Geometry: final body of the model. Coordinates: model frame, mm. A direction names the side the tool comes from. Give positions to 0.01 mm unless a question says otherwise; leave off trailing zeros. Order: outer loops, then holes, each group sorted by start corner. A loop starts at its lowest first (then second) coordinate and runs counter-clockwise, first axis right, second up. Notation, with made-up numbers: (-15.5, 0) -> (13.5, 0) arc R33 cw to (13.5, 32) -> close; hole circle Ø11 at (-40, 33.5). An arc over 180 degrees is marked (long way). Answer in a Markdown table with one row per item. Add a question column.
Q1. Line query: line 1 along Y through (x, z) = (-23, 0); line 2 along X through (y, z) = (28.5, 13.5); line 3 along Y through (x, z) = (-21.5, -3.5). Output: solid intervals per line, ascending. Write a range as from..to.
Q2. Contact query for flat-ended pins moving along their axis: P1, Ø10.5, axis at y = 55, z = 0.25, coming from the -X side; P2, Ø4.5, axis at x = 1, y = 52, coming from the -Z side; P3, Ø3, axis at x = 22.5, y = 14.5, coming from the -Z side; P4, Ø5.5, axis at y = 35.79, z = 0.25, coming from the +X side. Output: stop coordinate, or through.
Q3. Cut plane D-D on x = -10. Return the cut outline in (y, z), and give its area (3 significant figures).
Q4. Cut plane A-A on x = 0. Return the cut outline in (y, z), and give its area (3 significant figures).
Q5. Cut plane C-C on z = -16. Return the cut outline in (x, y).
Q6. Cut plane B-B on y = 20. Return the cut outline in (x, z), and give its area (3 significant figures).
Q7. Pull-direction query (Z, two-part tool) for faces 6 (the face through (-24.278, 48.132, -1.275)), 7 (the face through (23, 26.5, -7)), 8 (the face through (23, 47, -19.75)); classes: +Z half, -Z half, draft (parallel to the pull), parting line (faces both ways), or undercut.
Q8. Set-up query: faces 1 (the face through (22.25, 55, 5)), 2 (the face through (20.25, 42, 0)), 3 (the face through (-22.25, 55, 5)), 4 (the face through (23.21, 25, 8.82)), 5 (the face through (0, 51, 22.35)). Return all of +Z, -Z, +X, -X, +Y, -Y with unobstructed straight access to the full face (end or side cutting, diameter ignored); none if empty.
from build123d import *

# Parameters (mm, degrees)
BOSS_EXTRUDE1_DEPTH           = 70
SKETCH8_R                     = 4.5
CUT_EXTRUDE4_DEPTH            = 53.5
SKETCH10_R                    = 7.035
CUT_EXTRUDE5_DEPTH            = 4
FILLET13_R                    = 1
M8_CLEARANCE_HOLE1_AT_2_COUNT = 2
M8_CLEARANCE_HOLE1_AT_2_PITCH = 24.109474775
CUT_EXTRUDE6_REACH            = 54.5
SKETCH21_W                    = 30
SKETCH21_H                    = 26.5
M8_CLEARANCE_HOLE2_D          = 9
FILLET14_R                    = 5
SKETCH24_W                    = 10
SKETCH24_H                    = 38
CUT_EXTRUDE7_DEPTH            = 2.1
FILLET15_R                    = 0.5


with BuildPart() as part:
    # Sketch1 → Boss-Extrude1 (new body)
    with BuildSketch(Plane(origin=(0, 0, 0), x_dir=(1, 0, 0), z_dir=(0, 1, 0))):
        Polygon((-26.25, -26.25), (26.25, -26.25), (26.25, 19.75), (20.25, 19.75), (20.25, -20.25), (-20.25, -20.25), (-20.25, 19.75), (-26.25, 19.75), align=None)
    extrude(amount=BOSS_EXTRUDE1_DEPTH)

    # Sketch8 → Cut-Extrude4 (cut, through all)
    with BuildSketch(Plane(origin=(26.25, 0, 0), x_dir=(0, 0, -1), z_dir=(1, 0, 0))):
        with Locations((-0.25, 55)):
            Circle(SKETCH8_R)
    extrude(amount=-CUT_EXTRUDE4_DEPTH, mode=Mode.SUBTRACT)

    # Sketch10 → Cut-Extrude5 (cut)
    with BuildSketch(Plane.ZY.offset(26.25)):
        with Locations((0.25, 55)):
            Circle(SKETCH10_R)
    cut_extrude5 = extrude(amount=-CUT_EXTRUDE5_DEPTH, mode=Mode.SUBTRACT)

    # Mirror1: Cut-Extrude5 across plane
    add(cut_extrude5.mirror(Plane(origin=(0, 0, 0), x_dir=(0, 0, 1), z_dir=(1, 0, 0))), mode=Mode.SUBTRACT)

    # Fillet13
    fillet13_edges = [part.edges().sort_by_distance(p)[0] for p in [
        (26.25, 0, 3.25),
        (0, 0, 26.25),
        (0, 70, 20.25),
        (-26.25, 0, 3.25),
        (-23.25, 0, -19.75),
        (-20.25, 0, 0.25),
        (0, 0, 20.25),
        (20.25, 0, 0.25),
        (-20.25, 70, 0.25),
        (20.25, 35, -19.75),
        (26.25, 35, -19.75),
        (26.25, 35, 26.25),
        (-26.25, 35, 26.25),
        (-26.25, 35, -19.75),
        (-20.25, 35, -19.75),
        (-23.25, 70, -19.75),
        (-26.25, 70, 3.25),
        (0, 70, 26.25),
        (26.25, 70, 3.25),
        (23.25, 70, -19.75),
        (20.25, 70, 0.25),
        (23.25, 0, -19.75),
    ]]
    fillet(fillet13_edges, radius=FILLET13_R)

    # Sketch18 → M8 Clearance Hole1 (revolve, cut)
    with BuildSketch(Plane(origin=(-20.25, 35.786178525, 0.25), x_dir=(0, 0, -1), z_dir=(0, 1, 0))):
        Polygon((0, 0), (0, 15.703872786), (4.5, 13), (4.5, 0.025), (4.525, 0), align=None)
    m8_clearance_hole1 = revolve(axis=Axis((-13.9, 35.786178525, 0.25), (-1, 0, 0)), mode=Mode.SUBTRACT)

    # M8 Clearance Hole1 at 2: M8 Clearance Hole1 ×2
    with Locations(*[(0, -i * M8_CLEARANCE_HOLE1_AT_2_PITCH, 0) for i in range(1, M8_CLEARANCE_HOLE1_AT_2_COUNT)]):
        add(m8_clearance_hole1, mode=Mode.SUBTRACT)

    # Mirror2: M8 Clearance Hole1 across plane
    add(m8_clearance_hole1.mirror(Plane(origin=(0, 0, 0), x_dir=(0, 0, 1), z_dir=(1, 0, 0))), mode=Mode.SUBTRACT)

    # Mirror2 copy 1 sketch → Mirror2 copy 1 (revolve, cut)
    with BuildSketch(Plane(origin=(20.25, 11.676703751, 0.25), x_dir=(0, 0, -1), z_dir=(0, 1, 0))):
        Polygon((0, 0), (0, -15.703872786), (4.5, -13), (4.5, -0.025), (4.525, 0), align=None)
    revolve(axis=Axis((13.9, 11.676703751, 0.25), (-1, 0, 0)), mode=Mode.SUBTRACT)

    # Sketch21 → Cut-Extrude6 (cut, up to next)
    with BuildSketch(Plane.ZY.offset(-26.25), mode=Mode.PRIVATE) as cut_extrude6_sk1:
        with Locations((-4.75, 13.25)):
            Rectangle(SKETCH21_W, SKETCH21_H)
    cut_extrude6_tool1 = extrude(cut_extrude6_sk1.sketch, amount=CUT_EXTRUDE6_REACH, mode=Mode.PRIVATE) & part.part
    add(cut_extrude6_tool1.solids().sort_by_distance((26.25, 13.25, -4.75))[0], mode=Mode.SUBTRACT)

    # M8 Clearance Hole2 (through all)
    with Locations(Plane.XY.offset(26.25)):
        with Locations((0, 20)):
            Hole(M8_CLEARANCE_HOLE2_D / 2)

    # Fillet14
    fillet14_edges = [part.edges().sort_by_distance(p)[0] for p in [
        (23.25, 26.5, 10.25),
    ]]
    fillet(fillet14_edges, radius=FILLET14_R)

    # Sketch24 → Cut-Extrude7 (cut)
    with BuildSketch(Plane(origin=(0, 0, 20.25), x_dir=(-1, 0, 0), z_dir=(0, 0, -1))):
        with Locations((0, 51)):
            Rectangle(SKETCH24_W, SKETCH24_H)
    extrude(amount=-CUT_EXTRUDE7_DEPTH, mode=Mode.SUBTRACT)

    # Fillet15
    fillet15_edges = [part.edges().sort_by_distance(p)[0] for p in [
        (5, 69.707106781, 20.542893219),
        (-5, 69.707106781, 20.542893219),
        (5, 70, 21.8),
        (0, 70, 22.35),
        (5, 50.5, 20.25),
        (0, 32, 20.25),
        (-5, 50.5, 20.25),
        (-5, 51, 22.35),
        (-5, 70, 21.8),
        (0, 32, 22.35),
        (-5, 32, 21.3),
        (5, 51, 22.35),
        (5, 32, 21.3),
    ]]
    fillet(fillet15_edges, radius=FILLET15_R)


solid = part.part
Completed:
| question | item | result |
|---|---|---|
| 1 | line 1 | y = 0..7.18, 16.17..31.29, 40.28..47.97, 62.03..70 |
| 1 | line 2 | x = -26.25..-20.25, 20.25..26.25 |
| 1 | line 3 | y = 0..9.19, 14.16..33.3, 38.27..52.51, 57.49..70 |
| 2 | P1 | stops at x = -22.25 |
| 2 | P2 | stops at z = 22.35 |
| 2 | P3 | stops at z = 10.25 |
| 2 | P4 | passes through |
| 3 | outline | (0, 21.25) arc R1 ccw to (1, 20.25) -> (69, 20.25) arc R1 ccw to (70, 21.25) -> (70, 25.25) arc R1 ccw to (69, 26.25) -> (1, 26.25) arc R1 ccw to (0, 25.25) -> close |
| 3 | area | 419 mm² |
| 4 | outline | (0, 21.25) arc R1 ccw to (1, 20.25) -> (15.5, 20.25) -> (15.5, 26.25) -> (1, 26.25) arc R1 ccw to (0, 25.25) -> close; (24.5, 20.25) -> (31.5, 20.25) arc R0.5 ccw to (32, 20.75) -> (32, 21.85) arc R0.5 cw to (32.5, 22.35) -> (69.5, 22.35) arc R0.5 ccw to (70, 22.85) -> (70, 25.25) arc R1 ccw to (69, 26.25) -> (24.5, 26.25) -> close |
| 4 | area | 286 mm² |
| 5 | outline | (-26.25, 1) arc R1 ccw to (-25.25, 0) -> (-21.25, 0) arc R1 ccw to (-20.25, 1) -> (-20.25, 69) arc R1 ccw to (-21.25, 70) -> (-25.25, 70) arc R1 ccw to (-26.25, 69) -> close; (20.25, 26.5) -> (26.25, 26.5) -> (26.25, 69) arc R1 ccw to (25.25, 70) -> (21.25, 70) arc R1 ccw to (20.25, 69) -> close |
| 6 | outline | (-26.25, -18.75) arc R1 ccw to (-25.25, -19.75) -> (-21.25, -19.75) arc R1 ccw to (-20.25, -18.75) -> (-20.25, 20.25) -> (-4.5, 20.25) -> (-4.5, 26.25) -> (-25.25, 26.25) arc R1 ccw to (-26.25, 25.25) -> close; (4.5, 20.25) -> (20.25, 20.25) -> (20.25, 10.25) -> (26.25, 10.25) -> (26.25, 25.25) arc R1 ccw to (25.25, 26.25) -> (4.5, 26.25) -> close |
| 6 | area | 560 mm² |
| 7 | face 6 | undercut |
| 7 | face 7 | draft |
| 7 | face 8 | -Z half |
| 8 | face 1 | +X |
| 8 | face 2 | -Z, +Y, -Y |
| 8 | face 3 | -X |
| 8 | face 4 | -Z, +X, -Y |
| 8 | face 5 | -Z, +Y |
